```python
from build123d import *

# Parameters (mm, degrees)
SKETCH_1_W          = 96.5
SKETCH_1_H          = 18
SKETCH_1_W_2        = 92.5
SKETCH_1_H_2        = 14
EXTRUDE_1_DEPTH     = 6
FILLET_1_R          = 2
CHAMFER_1_SIZE      = 0.6
SKETCH_2_W          = 6
SKETCH_2_H          = 2
EXTRUDE_2_DEPTH     = 5.4
SKETCH_3_R          = 1.2
CUT_EXTRUDE_1_DEPTH = 52.846528331
SKETCH_4_R          = 2.05
CUT_EXTRUDE_2_DEPTH = 2
CUT_EXTRUDE_START   = -16
SKETCH_4_2_R        = 2.05
CUT_EXTRUDE_3_DEPTH = 2
CHAMFER_2_SIZE      = 0.6


with BuildPart() as part:
    # 草图1 → 凸台-拉伸1 (new body)
    with BuildSketch(Plane.XY):
        Rectangle(SKETCH_1_W, SKETCH_1_H)
        Rectangle(SKETCH_1_W_2, SKETCH_1_H_2, mode=Mode.SUBTRACT)
    extrude(amount=EXTRUDE_1_DEPTH)

    # 圆角1
    fillet_1_edges = [part.edges().sort_by_distance(p)[0] for p in [
        (48.25, -9, 3),
        (-48.25, -9, 3),
        (-48.25, 9, 3),
        (48.25, 9, 3),
    ]]
    fillet(fillet_1_edges, radius=FILLET_1_R)

    # 倒角1
    chamfer_1_edges = [part.edges().sort_by_distance(p)[0] for p in [
        (0, 7, 0),
        (-46.25, 0, 0),
        (0, -7, 0),
        (46.25, 0, 0),
    ]]
    chamfer(chamfer_1_edges, length=CHAMFER_1_SIZE)

    # 草图2 → 凸台-拉伸2 (add)
    with BuildSketch(Plane.XY.offset(6)):
        with Locations((-18.25, 6)):
            Rectangle(SKETCH_2_W, SKETCH_2_H)
        with Locations((-18.25, -6)):
            Rectangle(SKETCH_2_W, SKETCH_2_H)
        with Locations((18.25, 6)):
            Rectangle(SKETCH_2_W, SKETCH_2_H)
        with Locations((18.25, -6)):
            Rectangle(SKETCH_2_W, SKETCH_2_H)
    extrude(amount=-EXTRUDE_2_DEPTH)

    # 草图3 → 切除-拉伸1 (cut, through all)
    with BuildSketch(Plane(origin=(0, 9, 0), x_dir=(1, 0, 0), z_dir=(0, 1, 0))):
        with Locations(Location((-18.25, -3, 0), (0, 0, 270))):
            Circle(SKETCH_3_R)
        with Locations(Location((18.25, -3, 0), (0, 0, 270))):
            Circle(SKETCH_3_R)
    extrude(amount=-CUT_EXTRUDE_1_DEPTH, mode=Mode.SUBTRACT)

    # 草图4 → 切除-拉伸2 (cut)
    with BuildSketch(Plane(origin=(0, 9, 0), x_dir=(1, 0, 0), z_dir=(0, 1, 0))):
        with Locations(Location((-18.25, -3, 0), (0, 0, 270))):
            Circle(SKETCH_4_R)
        with Locations(Location((18.25, -3, 0), (0, 0, 270))):
            Circle(SKETCH_4_R)
    extrude(amount=-CUT_EXTRUDE_2_DEPTH, mode=Mode.SUBTRACT)

    # 草图4<2> → 切除-拉伸3 (cut)
    with BuildSketch(Plane(origin=(0, 9, 0), x_dir=(1, 0, 0), z_dir=(0, 1, 0)).offset(CUT_EXTRUDE_START)):
        with Locations(Location((-18.25, -3, 0), (0, 0, 270))):
            Circle(SKETCH_4_2_R)
        with Locations(Location((18.25, -3, 0), (0, 0, 270))):
            Circle(SKETCH_4_2_R)
    extrude(amount=-CUT_EXTRUDE_3_DEPTH, mode=Mode.SUBTRACT)

    # 倒角2
    chamfer_2_edges = [part.edges().sort_by_distance(p)[0] for p in [
        (0, -9, 6),
        (-48.25, 0, 6),
        (48.25, 0, 6),
        (0, 9, 6),
        (-47.664213562, 8.414213562, 6),
        (47.664213562, 8.414213562, 6),
        (47.664213562, -8.414213562, 6),
        (-47.664213562, -8.414213562, 6),
    ]]
    chamfer(chamfer_2_edges, length=CHAMFER_2_SIZE)


solid = part.part
```
Geometry check sheet. Reference: the model listing, model coordinates, mm. A direction names the side the tool comes from. Round coordinates to 2 decimals unless told otherwise and drop trailing zeros. Loops run counter-clockwise (first coordinate to the right, second up) from the corner with the lowest first, then second, coordinate; pieces in that order, holes last. Notation, with made-up numbers: (4.25, 57) - (51.25, 57) arc R14 cw to (51.25, 66) - close; hole circle Ø6 at (-14, -7.75). An arc over 180 degrees is marked (long way). Use a Markdown table: item, result.
Q1. Draft check along Z on faces 4 (the flat face through (34, -7, 3)), 5 (the conical face through (47.389, -8.165, 5.771)), 6 (the flat face through (-20, -7, 3)), 7 (the cylindrical face through (18.866, -7.986, 4.955)). Enter one of: released by +Z, released by -Z, zero draft, split by the parting line, or undercut.
Solutions:
| item | result |
|---|---|
| face 4 | zero draft |
| face 5 | released by +Z |
| face 6 | undercut |
| face 7 | undercut |
Q2. Material ranges on line 1 (X direction, y = 6.5, z = 3); line 2 (X direction, y = -4.25, z = 1.6); line 3 (X direction, y = -5.25, z = 2.5), recorded low to high.
Solutions:
| item | result |
|---|---|
| line 1 | x = -48.25 to -46.25, -21.25 to -19.45, -17.05 to -15.25, 15.25 to 17.05, 19.45 to 21.25, 46.25 to 48.25 |
| line 2 | x = -48.25 to -46.25, 46.25 to 48.25 |
| line 3 | x = -48.25 to -46.25, -21.25 to -19.34, -17.16 to -15.25, 15.25 to 17.16, 19.34 to 21.25, 46.25 to 48.25 |
Q3. Cross-section at A-A on x = -18.25. State how many separate pieces and enclosed holes the cut face has, plus the area to 3 significant figures.
Solutions:
| item | result |
|---|---|
| separate pieces | 4 |
| enclosed holes | 0 |
| area | 18.9 mm2 |
Q4. Cross-section at C-C on y = 0.75. Record the cut outline in (x, z), plus the area to 3 significant figures.
Solutions:
| item | result |
|---|---|
| outline | (-48.25, 0) - (-46.85, 0) - (-46.25, 0.6) - (-46.25, 6) - (-47.65, 6) - (-48.25, 5.4) - close; (46.25, 0.6) - (46.85, 0) - (48.25, 0) - (48.25, 5.4) - (47.65, 6) - (46.25, 6) - close |
| area | 23.3 mm2 |
Q5. Access from +Z, -Z, +X, -X, +Y, -Y to the whole of each face (thin tool, end or side, straight path). Record for faces 1 (the flat face through (18, -6, 0.6)), 2 (the flat face through (0, 7, 3)), 3 (the cylindrical face through (47.65, 8.43, 2.74)).
Solutions:
| item | result |
|---|---|
| face 1 | -Z |
| face 2 | +Z, -Z |
| face 3 | +Z, -Z, +X, +Y |
Q6. Go/stop test with flat-tipped pins: P1, Ø3, axis at x = 18.25, z = 3, coming from the +Y side; P2, Ø0.6, axis at x = 18, y = -6, coming from the -Z side; P3, Ø2, axis at x = -17.5, y = -6.5, coming from the -Z side. Record where each tip stops, or that it passes through.
Solutions:
| item | result |
|---|---|
| P1 | stops at y = 7 |
| P2 | stops at z = 0.6 |
| P3 | stops at z = 0.1 |
Q7. Cross-section at B-B on x = 29. Record the cut outline in (y, z).
Solutions:
| item | result |
|---|---|
| outline | (-9, 0) - (-7.6, 0) - (-7, 0.6) - (-7, 6) - (-8.4, 6) - (-9, 5.4) - close; (7, 0.6) - (7.6, 0) - (9, 0) - (9, 5.4) - (8.4, 6) - (7, 6) - close |
